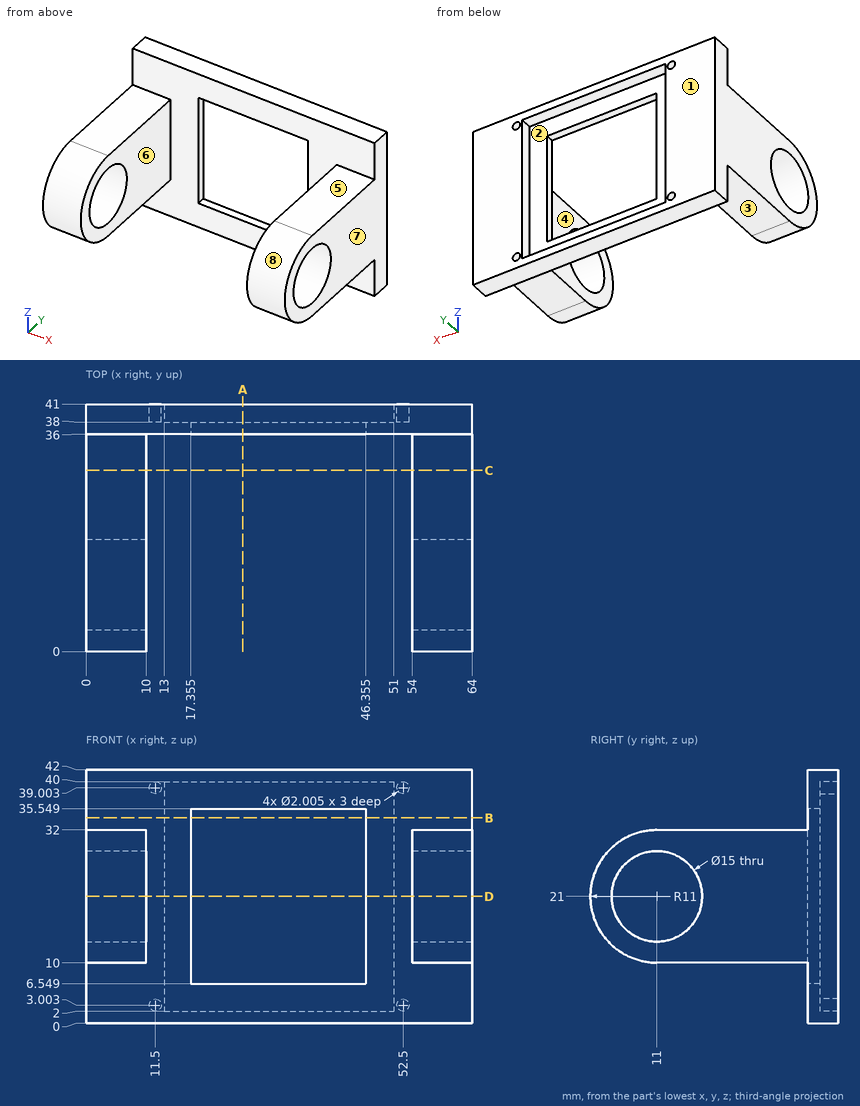
Answer from the drawing. Dimensions are ordinates in mm from the lowest x, y and z of the part. A direction names the side the tool comes from. Round coordinates to 2 decimals unless told otherwise and drop trailing zeros. Loops run counter-clockwise (first coordinate to the right, second up) from the corner with the lowest first, then second, coordinate; pieces in that order, holes last. Notation, with made-up numbers: (57.5, -5) - (87.5, -5) arc R32 cw to (87.5, 30) - close; hole circle Ø7 at (16.5, 41.25). An arc over 180 degrees is marked (long way). Return JSON: item names as keys, results as strings. Group by question number.
1. Which of the six approach directions +Z, -Z, +X, -X, +Y, -Y give full straight-line access (tool end or side, diameter ignored) to the marked faces 1, 2, 3, 4 and 5?
2. The part is cut by section A-A on x = 26. Determine the outline of the cut face in (y, z).
3. The part is cut by section B-B on z = 34. Determine the outline of the cut face in (x, y) (1 decimal), then the cut area to 3 significant figures.
4. The mould has two halves that part along X. Classify the marked faces 6, 7 and 8: pulls with the +X half, pulls with the -X half, needs draft (parallel to the pull), parting line crosses it, or undercut.
5. The part is cut by section C-C on y = 30. Determine the outline of the cut face in (x, z).
6. The part is cut by section D-D on z = 21. Determine the outline of the cut face in (x, y) (1 decimal), then the cut area to 3 significant figures.
7. Consider probe 1 along X at (y, z) = (26, 15); probe 2 along X at (y, z) = (38.5, 4.5); probe 3 along Y at (x, z) = (60, 21). Determine where each line is inside the solid, lowest interval first.
8. Each of these flat-tipped pins is pushed along its axis until it touches: P1, Ø4, axis at x = 22.5, z = 38, coming from the -Y side; P2, Ø5, axis at x = 5, y = 24, coming from the +Z side; P3, Ø19, axis at x = 26.5, z = 24, coming from the +Y side. Where does it stop, or does it pass through?
Resolved:
{
 "1": {"face 1": "+Z, -Z, +X, -X, +Y", "face 2": "+Y", "face 3": "-Z, +X, -X, -Y", "face 4": "+Z, -Z, -Y", "face 5": "+Z, +X, -X, -Y"},
 "2": {"outline": "(36, 0) - (41, 0) - (41, 2) - (38, 2) - (38, 6.55) - (36, 6.55) - close; (36, 35.55) - (38, 35.55) - (38, 40) - (41, 40) - (41, 42) - (36, 42) - close"},
 "3": {"outline": "(0, 36) - (17.4, 36) - (17.4, 38) - (13, 38) - (13, 41) - (0, 41) - close; (46.4, 36) - (64, 36) - (64, 41) - (51, 41) - (51, 38) - (46.4, 38) - close", "area": "148 mm²"},
 "4": {"face 6": "undercut", "face 7": "pulls with the +X half", "face 8": "needs draft"},
 "5": {"outline": "(0, 10) - (10, 10) - (10, 32) - (0, 32) - close; (54, 10) - (64, 10) - (64, 32) - (54, 32) - close"},
 "6": {"outline": "(0, 0) - (10, 0) - (10, 3.5) - (0, 3.5) - close; (0, 18.5) - (10, 18.5) - (10, 36) - (17.4, 36) - (17.4, 38) - (13, 38) - (13, 41) - (0, 41) - close; (46.4, 36) - (54, 36) - (54, 18.5) - (64, 18.5) - (64, 41) - (51, 41) - (51, 38) - (46.4, 38) - close; (54, 0) - (64, 0) - (64, 3.5) - (54, 3.5) - close", "area": "568 mm²"},
 "7": {"probe 1": "x = 0 to 10, 54 to 64", "probe 2": "x = 0 to 13, 51 to 64", "probe 3": "y = 0 to 3.5, 18.5 to 41"},
 "8": {"P1": "stops at y = 36", "P2": "stops at z = 32", "P3": "stops at y = 38"}
}
